```python
from build123d import *

# Parameters (mm, degrees)
SKETCH1_W           = 708
SKETCH1_H           = 120
BOSS_EXTRUDE1_DEPTH = 4
CUT_EXTRUDE1_REACH  = 720.109
SKETCH2_R           = 2.55
SKETCH2_W           = 30
SKETCH2_H           = 48
SKETCH5_R           = 2.6
CUT_EXTRUDE3_DEPTH  = 10
SKETCH6_R           = 2.6
CUT_EXTRUDE4_DEPTH  = 10


with BuildPart() as part:
    # Sketch1 → Boss-Extrude1 (new body)
    with BuildSketch(Plane.XY):
        with Locations((354, 60)):
            Rectangle(SKETCH1_W, SKETCH1_H)
    extrude(amount=BOSS_EXTRUDE1_DEPTH)

    # Sketch2 → Cut-Extrude1 (cut, up to next)
    with BuildSketch(Plane.XY.offset(4), mode=Mode.PRIVATE) as cut_extrude1_sk1:
        with Locations((623, 34)):
            Circle(SKETCH2_R)
    cut_extrude1_tool1 = extrude(cut_extrude1_sk1.sketch, amount=-CUT_EXTRUDE1_REACH, mode=Mode.PRIVATE) & part.part
    # Sketch2 → Cut-Extrude1 (cut, up to next)
    with BuildSketch(Plane.XY.offset(4), mode=Mode.PRIVATE) as cut_extrude1_sk2:
        with Locations((663, 34)):
            Circle(SKETCH2_R)
    cut_extrude1_tool2 = extrude(cut_extrude1_sk2.sketch, amount=-CUT_EXTRUDE1_REACH, mode=Mode.PRIVATE) & part.part
    # Sketch2 → Cut-Extrude1 (cut, up to next)
    with BuildSketch(Plane.XY.offset(4), mode=Mode.PRIVATE) as cut_extrude1_sk3:
        with Locations((643, 34)):
            Rectangle(SKETCH2_W, SKETCH2_H)
    cut_extrude1_tool3 = extrude(cut_extrude1_sk3.sketch, amount=-CUT_EXTRUDE1_REACH, mode=Mode.PRIVATE) & part.part
    add(cut_extrude1_tool1.solids().sort_by_distance((623, 34, 4))[0], mode=Mode.SUBTRACT)
    add(cut_extrude1_tool2.solids().sort_by_distance((663, 34, 4))[0], mode=Mode.SUBTRACT)
    add(cut_extrude1_tool3.solids().sort_by_distance((643, 34, 4))[0], mode=Mode.SUBTRACT)

    # Sketch5 → Cut-Extrude3 (cut)
    with BuildSketch(Plane(origin=(0, 0, 0), x_dir=(-1, 0, 0), z_dir=(0, 0, -1))):
        with Locations((-694, 105)):
            Circle(SKETCH5_R)
        with Locations((-14, 105)):
            Circle(SKETCH5_R)
    extrude(amount=-CUT_EXTRUDE3_DEPTH, mode=Mode.SUBTRACT)

    # Sketch6 → Cut-Extrude4 (cut)
    with BuildSketch(Plane(origin=(0, 0, 0), x_dir=(-1, 0, 0), z_dir=(0, 0, -1))):
        with Locations((-694, 20)):
            Circle(SKETCH6_R)
    cut_extrude4 = extrude(amount=-CUT_EXTRUDE4_DEPTH, mode=Mode.SUBTRACT)

    # Mirror7: Cut-Extrude4 across plane
    add(cut_extrude4.mirror(Plane(origin=(354, 0, 0), x_dir=(0, 0, 1), z_dir=(1, 0, 0))), mode=Mode.SUBTRACT)


solid = part.part
```
Verification items for the finished model (mm, model axes). Coordinates: 2 decimals unless noted, no trailing zeros. Loops run counter-clockwise (first coordinate to the right, second up) from the corner with the lowest first, then second, coordinate; pieces in that order, holes last. Notation, with made-up numbers: (44, -13.5) -> (53, -13.5) arc R24 ccw to (53, 8.5) -> close; hole circle Ø3 at (-30.5, 70). An arc over 180 degrees is marked (long way). Answer in a Markdown table with one row per item. Add a question column.
1. Depth check by flat-ended pin: P1, Ø3, axis at x = 694, y = 20, coming from the +Z side. Enter the tip coordinate at first touch or a pass-through.
2. Material ranges on probe 1 along Y at (x, z) = (694, 2.95); probe 2 along X at (y, z) = (105.5, 0.7); probe 3 along X at (y, z) = (42, 2.9), recorded low to high. Write a range as [from, to].
3. Section check A-A, the plane z = 3.05. Enter the section's corners in (x, y).
Derived:
| question | item | result |
|---|---|---|
| 1 | P1 | passes through |
| 2 | probe 1 | y = [0, 17.4], [22.6, 102.4], [107.6, 120] |
| 2 | probe 2 | x = [0, 11.45], [16.55, 691.45], [696.55, 708] |
| 2 | probe 3 | x = [0, 628], [658, 708] |
| 3 | outline | (0, 0) -> (708, 0) -> (708, 120) -> (0, 120) -> close; hole circle Ø5.2 at (14, 20); hole circle Ø5.2 at (14, 105); hole circle Ø5.1 at (623, 34); hole (628, 10) -> (658, 10) -> (658, 58) -> (628, 58) -> close; hole circle Ø5.1 at (663, 34); hole circle Ø5.2 at (694, 20); hole circle Ø5.2 at (694, 105) |
